from build123d import *

# Parameters (mm, degrees)
SKETCH_1_W          = 80
SKETCH_1_H          = 50
SKETCH_1_R          = 2.1
SKETCH_1_W_2        = 44.8
SKETCH_1_H_2        = 28
EXTRUDE_1_DEPTH     = 5
FILLET_1_R          = 2
SKETCH_2_W          = 48.8
SKETCH_2_H          = 30.5
SKETCH_2_W_2        = 44.8
SKETCH_2_H_2        = 28
EXTRUDE_2_DEPTH     = 20
SKETCH_3_W          = 48.8
SKETCH_3_H          = 30.5
SKETCH_3_R          = 6.6
EXTRUDE_3_DEPTH     = 3
FILLET_2_R          = 2
SKETCH_4_R          = 1.6
CUT_EXTRUDE_1_DEPTH = 55.854352608


with BuildPart() as part:
    # 草图1 → 凸台-拉伸1 (new body)
    with BuildSketch(Plane(origin=(0, 0, 0), x_dir=(1, 0, 0), z_dir=(0, 1, 0))):
        Rectangle(SKETCH_1_W, SKETCH_1_H)
        with Locations(Location((35, 20, 0), (0, 0, 270))):
            Circle(SKETCH_1_R, mode=Mode.SUBTRACT)
        with Locations(Location((35, -20, 0), (0, 0, 90))):
            Circle(SKETCH_1_R, mode=Mode.SUBTRACT)
        with Locations(Location((-35, -20, 0), (0, 0, 270))):
            Circle(SKETCH_1_R, mode=Mode.SUBTRACT)
        with Locations(Location((-35, 20, 0), (0, 0, 90))):
            Circle(SKETCH_1_R, mode=Mode.SUBTRACT)
        Rectangle(SKETCH_1_W_2, SKETCH_1_H_2, mode=Mode.SUBTRACT)
    extrude(amount=EXTRUDE_1_DEPTH)

    # 圆角1
    fillet_1_edges = [part.edges().sort_by_distance(p)[0] for p in [
        (40, 2.5, 25),
        (-40, 2.5, 25),
        (-40, 2.5, -25),
        (40, 2.5, -25),
    ]]
    fillet(fillet_1_edges, radius=FILLET_1_R)

    # 草图2 → 凸台-拉伸2 (add)
    with BuildSketch(Plane(origin=(0, 5, 0), x_dir=(1, 0, 0), z_dir=(0, 1, 0))):
        Rectangle(SKETCH_2_W, SKETCH_2_H)
        Rectangle(SKETCH_2_W_2, SKETCH_2_H_2, mode=Mode.SUBTRACT)
    extrude(amount=EXTRUDE_2_DEPTH)

    # 草图3 → 凸台-拉伸3 (add)
    with BuildSketch(Plane(origin=(0, 25, 0), x_dir=(1, 0, 0), z_dir=(0, 1, 0))):
        Rectangle(SKETCH_3_W, SKETCH_3_H)
        with Locations(Location((0, 0, 0), (0, 0, 270))):
            Circle(SKETCH_3_R, mode=Mode.SUBTRACT)
    extrude(amount=EXTRUDE_3_DEPTH)

    # 圆角2
    fillet_2_edges = [part.edges().sort_by_distance(p)[0] for p in [
        (24.4, 16.5, 15.25),
        (24.4, 16.5, -15.25),
        (-24.4, 16.5, -15.25),
        (-24.4, 16.5, 15.25),
    ]]
    fillet(fillet_2_edges, radius=FILLET_2_R)

    # 草图4 → 切除-拉伸1 (cut, through all)
    with BuildSketch(Plane(origin=(0, 28, 0), x_dir=(1, 0, 0), z_dir=(0, 1, 0))):
        with Locations(Location((0, -9.5, 0), (0, 0, 270))):
            Circle(SKETCH_4_R)
        with Locations(Location((-8.227241336, 4.75, 0), (0, 0, 270))):
            Circle(SKETCH_4_R)
        with Locations(Location((8.227241336, 4.75, 0), (0, 0, 270))):
            Circle(SKETCH_4_R)
    extrude(amount=-CUT_EXTRUDE_1_DEPTH, mode=Mode.SUBTRACT)


solid = part.part
For this review, take the finished solid that the model builds, in its own axes (mm). A direction names the side the tool comes from. Round coordinates to 2 decimals unless told otherwise and drop trailing zeros. Loops run counter-clockwise (first coordinate to the right, second up) from the corner with the lowest first, then second, coordinate; pieces in that order, holes last. Notation, with made-up numbers: (0, -2.75) - (30, -2.75) arc R18 cw to (30, 26.25) - close; hole circle Ø3 at (-6, 49). An arc over 180 degrees is marked (long way). Put each result on its own line as item: value. Start each with the question number.
1. For probe 1 along X at (y, z) = (1.75, -20); probe 2 along X at (y, z) = (14.5, -6.5); probe 3 along X at (y, z) = (3.75, -4.5), list the stretches that pass through material, from the lowest coordinate up. Write a range as [from, to].
2. Consider section C-C on z = -20. State the section outline as (x, y) points.
3. Insertion check: P1, Ø5.5, axis at x = -35, z = -20, coming from the +Y side; P2, Ø4, axis at x = 4.5, z = -10.5, coming from the -Y side; P3, Ø8, axis at x = -28.5, y = 10.5, coming from the +Z side; P4, Ø4, axis at y = 13, z = 11.5, coming from the -X side. Each pin has a flat end and moves straight along its axis. Give the tip position at first contact, or say it passes through.
4. Consider section B-B on x = 0. State the section outline as (y, z) points, plus the area to 3 significant figures.
5. For faces 4 (the cylindrical face through (23.83, 16.34, -14.65)), 5 (the cylindrical face through (-23.83, 16.34, -14.65)), 6 (the flat face through (24.4, 16, 0)), 7 (the flat face through (22.4, 12, 0)), 8 (the flat face through (0, 16, 15.25)), list the 3-axis set-ups (+Z, -Z, +X, -X, +Y, -Y) from which the entire face can be reached by the end or side of a thin tool; tool diameter is ignored.
6. Consider section D-D on x = -17. State the section outline as (y, z) points.
7. Consider section A-A on z = 9.5. State the section outline as (x, y) points.
8. Mouldability with a two-part tool opening along Z and no side actions: class faces 1 (the flat face through (5, 25, -6)), 2 (the cylindrical face through (-23.83, 16.66, 14.65)), 3 (the cylindrical face through (39.4, 2.54, -24.43)) as +Z half, -Z half, draft (parallel to the pull), parting line (faces both ways), or undercut.
Result sheet:
1. probe 1: [-40, -37.1], [-32.9, 32.9], [37.1, 40]
1. probe 2: [-24.4, -22.4], [22.4, 24.4]
1. probe 3: [-40, -22.4], [22.4, 40]
2. outline: (-40, 0) - (-37.1, 0) - (-37.1, 5) - (-40, 5) - close; (-32.9, 0) - (32.9, 0) - (32.9, 5) - (-32.9, 5) - close; (37.1, 0) - (40, 0) - (40, 5) - (37.1, 5) - close
3. P1: y = 5
3. P2: y = 25
3. P3: through
3. P4: x = -24.4
4. outline: (0, -25) - (5, -25) - (5, -15.25) - (28, -15.25) - (28, -6.6) - (25, -6.6) - (25, -14) - (0, -14) - close; (0, 14) - (25, 14) - (25, 11.1) - (28, 11.1) - (28, 15.25) - (5, 15.25) - (5, 25) - (0, 25) - close; (25, 6.6) - (28, 6.6) - (28, 7.9) - (25, 7.9) - close
4. area: 202 mm^2
5. face 4: -Z, +X, +Y
5. face 5: -Z, -X, +Y
5. face 6: +Z, -Z, +X, +Y
5. face 7: -Y
5. face 8: +Z, +X, -X, +Y
6. outline: (0, -25) - (5, -25) - (5, -15.25) - (28, -15.25) - (28, 15.25) - (5, 15.25) - (5, 25) - (0, 25) - (0, 14) - (25, 14) - (25, -14) - (0, -14) - close
7. outline: (-40, 0) - (-22.4, 0) - (-22.4, 25) - (-1.6, 25) - (-1.6, 28) - (-24.4, 28) - (-24.4, 5) - (-40, 5) - close; (1.6, 25) - (22.4, 25) - (22.4, 0) - (40, 0) - (40, 5) - (24.4, 5) - (24.4, 28) - (1.6, 28) - close
8. face 1: undercut
8. face 2: +Z half
8. face 3: -Z half
